```python
from build123d import *

# Parameters (mm, degrees)
SKETCH1_R           = 2.159
BOSS_EXTRUDE1_DEPTH = 1.5875
SKETCH2_W           = 2.54
SKETCH2_H           = 3.81
CUT_EXTRUDE1_DEPTH  = 1.5875
FILLET1_R           = 2.54
FILLET2_R           = 2.54


with BuildPart() as part:
    # Sketch1 → Boss-Extrude1 (new body)
    with BuildSketch(Plane.XY):
        with BuildLine():
            Line((9.32893445, 30.396375958), (9.32893445, 18.483132928))
            Line((9.32893445, 18.483132928), (60.52106555, 18.483132928))
            Line((60.52106555, 18.483132928), (60.52106555, 30.396375958))
            ThreePointArc((60.52106555, 30.396375958), (67.725532775, 37.600843183), (74.93, 30.396375958))
            Line((74.93, 30.396375958), (74.93, 28.575))
            Line((74.93, 28.575), (69.85, 28.575))
            Line((69.85, 28.575), (69.85, 0))
            Line((69.85, 0), (53.975, 0))
            Line((53.975, 0), (53.975, 12.133132928))
            Line((53.975, 12.133132928), (15.875, 12.133132928))
            Line((15.875, 12.133132928), (15.875, 0))
            Line((15.875, 0), (0, 0))
            Line((0, 0), (0, 28.575))
            Line((0, 28.575), (-5.08, 28.575))
            Line((-5.08, 28.575), (-5.08, 30.396375958))
            ThreePointArc((-5.08, 30.396375958), (2.124467225, 37.600843183), (9.32893445, 30.396375958))
        make_face()
        with Locations((11.1125, 4.805875958)):
            Circle(SKETCH1_R, mode=Mode.SUBTRACT)
        with Locations((58.7375, 4.805875958)):
            Circle(SKETCH1_R, mode=Mode.SUBTRACT)
    extrude(amount=BOSS_EXTRUDE1_DEPTH)

    # Sketch2 → Cut-Extrude1 (cut)
    with BuildSketch(Plane.XY.offset(1.5875)):
        with Locations((5.51893445, 25.4)):
            Rectangle(SKETCH2_W, SKETCH2_H)
        with Locations((64.33106555, 25.4)):
            Rectangle(SKETCH2_W, SKETCH2_H)
    extrude(amount=-CUT_EXTRUDE1_DEPTH, mode=Mode.SUBTRACT)

    # Fillet1
    fillet1_edges = [part.edges().sort_by_distance(p)[0] for p in [
        (60.52106555, 18.483132928, 0.79375),
        (69.85, 28.575, 0.79375),
        (69.85, 0, 0.79375),
        (53.975, 0, 0.79375),
        (53.975, 12.133132928, 0.79375),
        (15.875, 12.133132928, 0.79375),
        (15.875, 0, 0.79375),
        (0, 0, 0.79375),
        (0, 28.575, 0.79375),
        (9.32893445, 18.483132928, 0.79375),
    ]]
    fillet(fillet1_edges, radius=FILLET1_R)

    # Fillet2
    fillet2_edges = [part.edges().sort_by_distance(p)[0] for p in [
        (-5.08, 28.575, 0.79375),
        (74.93, 28.575, 0.79375),
    ]]
    fillet(fillet2_edges, radius=FILLET2_R)


solid = part.part
```
The listing builds one solid part. Answer for the finished solid, in the listing's coordinates (mm). A direction names the side the tool comes from. Round coordinates to 2 decimals unless told otherwise and drop trailing zeros. Order: outer loops, then holes, each group sorted by start corner. A loop starts at its lowest first (then second) coordinate and runs counter-clockwise, first axis right, second up. Notation, with made-up numbers: (62.5, 65) - (89.5, 65) arc R18 cw to (89.5, 96) - close; hole circle Ø5 at (76.5, -25). An arc over 180 degrees is marked (long way). Put each result on its own line as item: value. Start each with the question number.
(1) Determine the mould class of faces 1 (the cylindrical face through (70.604, 27.841, 0.805)), 2 (the flat face through (6, 27.305, 1)), 3 (the flat face through (8, 0, 1)) for opening direction X: released by +X, released by -X, zero draft, split by the parting line, or undercut.
(2) Given P1, Ø0.5, axis at x = 64.5, z = 0.5, coming from the +Y side; P2, Ø0.5, axis at y = 6.5, z = 0.5, coming from the +X side; P3, Ø0.8, axis at y = 26.5, z = 0.5, coming from the +X side; P4, Ø1, axis at x = 25, y = 19.5, coming from the +Z side, each flat-ended and moving along its own axis, determine where each tip first touches the part or whether it passes through.
(3) Find section C-C (x = 49.5). Give the vertices of the cut face in (y, z).
(4) For faces 4 (the flat face through (64, 27.305, 1)), 5 (the cylindrical face through (59.76, 19.21, 0.8)), 6 (the cylindrical face through (15.111, 0.724, 0.805)), determine the directions among +Z, -Z, +X, -X, +Y, -Y from which every point of the face is accessible in a straight line to the end or side of a thin tool.
(5) Find section B-B (y = 3.5). State how many separate pieces and enclosed holes the cut face has, plus the area to 3 significant figures.
(6) Find section A-A (y = 35). Give the vertices of the cut face in (x, z), plus the area to 3 significant figures.
(7) Straight lines are drawn through the part: probe 1 along X at (y, z) = (24, 0.75); probe 2 along X at (y, z) = (3.5, 0.5) (3 decimals); probe 3 along Y at (x, z) = (26, 0.1). For each, find the intervals that lie inside material, in ascending order. Write a range as from..to.
Reply:
1. face 1: released by +X
1. face 2: undercut
1. face 3: zero draft
2. P1: y = 36.96
2. P2: x = 69.85
2. P3: x = 70
2. P4: through
3. outline: (12.13, 0) - (18.48, 0) - (18.48, 1.59) - (12.13, 1.59) - close
4. face 4: +Z, -Z
4. face 5: +Z, -Z, +Y
4. face 6: +Z, -Z, -Y
5. separate pieces: 4
5. enclosed holes: 0
5. area: 39.5 mm^2
6. outline: (-3.42, 0) - (7.67, 0) - (7.67, 1.59) - (-3.42, 1.59) - close; (62.18, 0) - (73.27, 0) - (73.27, 1.59) - (62.18, 1.59) - close
6. area: 35.2 mm^2
7. probe 1: 0..4.25, 6.79..9.33, 60.52..63.06, 65.6..69.85
7. probe 2: 0..9.393, 12.832..15.875, 53.975..57.018, 60.457..69.85
7. probe 3: 12.13..18.48
